CAD build for the part. Positions are in the model's coordinates, mm. Give positions to 0.01 mm unless a question says otherwise; leave off trailing zeros. Loops run counter-clockwise (first coordinate to the right, second up) from the corner with the lowest first, then second, coordinate; pieces in that order, holes last.
Item 1: Mould opens along X. For faces 1 (the cylindrical face through (-3, 0, 24)), 2 (the conical face through (-5.16, 0.11, 10.57)), 3 (the flat face through (-3, -3, 8)), 4 (the cylindrical face through (-1.73, 0.04, 7.81)) say: released by +X, released by -X, zero draft, split by the parting line, or undercut.
Item 2: Probe probe 1 along Z at (x, y) = (0, -0.2); probe 2 along X at (y, z) = (-0.3, 0); probe 3 along X at (y, z) = (-0.75, 1). List the from-to ranges inside material, lowest first.
Item 3: Saw through at C-C on z = 16. Give the cut face in (x, y).
Item 4: Drop flat-ended pins along their axis: P1, Ø3, axis at x = -4.5, y = -1, coming from the -Z side; P2, Ø1.5, axis at x = 6.5, y = 2, coming from the +Z side; P3, Ø4, axis at x = 7.5, z = 11, coming from the -Y side. Give the stop position or say it passes through.
Item 5: Saw through at A-A on y = 0. Give the cut face in (x, z).
Item 6: Saw through at D-D on z = 10. Give the cut face in (x, y), plus the area to 3 significant figures.
Item 7: Saw through at B-B on z = 0. Give the cut face in (x, y), plus the area to 3 significant figures.
from build123d import *

# Parameters (mm, degrees)
SZKIC1_W                        = 3
SZKIC1_H                        = 22
WYTNIJ_WYCI_GNI_CIE1_DEPTH      = 11
WYTNIJ_WYCI_GNI_CIE1_DEPTH_BACK = 11
SZKIC3_R                        = 8
WYTNIJ_WYCI_GNI_CIE2_DEPTH      = 4
WYTNIJ_WYCI_GNI_CIE2_DEPTH_BACK = 4
SFAZOWANIE1_SIZE                = 1.1


with BuildPart() as part:
    # Szkic1 → Obrót1 (revolve)
    with BuildSketch(Plane(origin=(0, 0, 0), x_dir=(1, 0, 0), z_dir=(0, 1, 0))):
        with BuildLine():
            Line((0, 10), (0, -14))
            Line((0, -14), (3, -14))
            Line((3, -14), (8.46133223, -5.329714522))
            ThreePointArc((8.46133223, -5.329714522), (8.754917053, 4.832331465), (0, 10))
        make_face()
        with Locations((1.5, -25)):
            Rectangle(SZKIC1_W, SZKIC1_H)
    revolve(axis=Axis((0, 0, -26.043516498), (0, 0, 1)))

    # Szkic2 → Wytnij-wyciągnięcie1 (cut, two sides)
    with BuildSketch(Plane(origin=(0, 0, 0), x_dir=(0, 0, -1), z_dir=(1, 0, 0))) as wytnij_wyci_gni_cie1_sk:
        with BuildLine():
            Line((-14, 3), (9.539392014, 3))
            ThreePointArc((9.539392014, 3), (3.447736008, 9.386858709), (-5.329714522, 8.46133223))
            Line((-5.329714522, 8.46133223), (-14, 3))
        make_face()
        with BuildLine():
            Line((-14, -3), (9.539392014, -3))
            ThreePointArc((9.539392014, -3), (3.447736008, -9.386858709), (-5.329714522, -8.46133223))
            Line((-5.329714522, -8.46133223), (-14, -3))
        make_face()
    extrude(amount=WYTNIJ_WYCI_GNI_CIE1_DEPTH, mode=Mode.SUBTRACT)
    extrude(wytnij_wyci_gni_cie1_sk.sketch, amount=-WYTNIJ_WYCI_GNI_CIE1_DEPTH_BACK, mode=Mode.SUBTRACT)

    # Szkic3 → Wytnij-wyciągnięcie2 (cut, two sides)
    with BuildSketch(Plane(origin=(0, 0, 0), x_dir=(1, 0, 0), z_dir=(0, 1, 0))) as wytnij_wyci_gni_cie2_sk:
        Circle(SZKIC3_R)
    extrude(amount=WYTNIJ_WYCI_GNI_CIE2_DEPTH, mode=Mode.SUBTRACT)
    extrude(wytnij_wyci_gni_cie2_sk.sketch, amount=-WYTNIJ_WYCI_GNI_CIE2_DEPTH_BACK, mode=Mode.SUBTRACT)

    # Sfazowanie1
    sfazowanie1_edges = [part.edges().sort_by_distance(p)[0] for p in [
        (-3, 0, 36),
    ]]
    chamfer(sfazowanie1_edges, length=SFAZOWANIE1_SIZE)


solid = part.part
Results below:
1. face 1: split by the parting line
1. face 2: released by -X
1. face 3: zero draft
1. face 4: undercut
2. probe 1: z = -10 to -8, 8 to 36
2. probe 2: x = -10 to -8, 8 to 10
2. probe 3: x = -9.92 to -7.94, 7.94 to 9.92
3. outline: circle Ø6 at (0, 0)
4. P1: stops at z = -9.5
4. P2: stops at z = 9.16
4. P3: passes through
5. outline: (-8.46, 5.33) arc R10 ccw (long way) to (8.46, 5.33) - (3, 14) - (3, 34.9) - (1.9, 36) - (-1.9, 36) - (-3, 34.9) - (-3, 14) - close; hole circle Ø16 at (0, 0)
6. outline: (-4.63, -3) - (4.63, -3) arc R5.52 ccw to (4.63, 3) - (-4.63, 3) arc R5.52 ccw to start
6. area: 62.8 mm2
7. outline: (-9.54, -3) - (-8, -3) - (-8, 3) - (-9.54, 3) arc R10 ccw to start; (8, -3) - (9.54, -3) arc R10 ccw to (9.54, 3) - (8, 3) - close
7. area: 22.2 mm2
